Model file for the job. Use its own axes, mm. Coordinates: 2 decimals unless noted, no trailing zeros. Order: outer loops, then holes, each group sorted by start corner. A loop starts at its lowest first (then second) coordinate and runs counter-clockwise, first axis right, second up. Notation, with made-up numbers: M 83,-32 L 124,-32 A18 cw 124,-16 Z; hole C -1,-13.75 d10. An arc over 180 degrees is marked long. Return JSON: item names as keys, results as strings.
```python
from build123d import *

# Parameters (mm, degrees)
SKETCH1_W           = 12.7
SKETCH1_H           = 80
BOSS_EXTRUDE1_DEPTH = 12.7
SKETCH2_R           = 2.5
SKETCH2_R_2         = 2
CUT_EXTRUDE1_DEPTH  = 13.7


with BuildPart() as part:
    # Sketch1 → Boss-Extrude1 (new body)
    with BuildSketch(Plane.XY):
        with Locations((6.35, 40)):
            Rectangle(SKETCH1_W, SKETCH1_H)
    extrude(amount=BOSS_EXTRUDE1_DEPTH)

    # Sketch2 → Cut-Extrude1 (cut, through all)
    with BuildSketch(Plane.XY):
        with Locations((6.35, 5)):
            Circle(SKETCH2_R)
        with Locations((6.35, 20)):
            Circle(SKETCH2_R)
        with Locations((6.35, 60)):
            Circle(SKETCH2_R_2)
        with Locations((6.35, 75)):
            Circle(SKETCH2_R_2)
    extrude(amount=CUT_EXTRUDE1_DEPTH, mode=Mode.SUBTRACT)


solid = part.part
```
Item 1: Saw through at A-A (y = 60). Write the cut outline in (x, z).
Check result:
{"outline": "M 0,0 L 4.35,0 L 4.35,12.7 L 0,12.7 Z; M 8.35,0 L 12.7,0 L 12.7,12.7 L 8.35,12.7 Z"}
Item 2: Saw through at B-B (z = 8.75). Write the cut outline in (x, y), and give its area (3 significant figures).
Check result:
{"outline": "M 0,0 L 12.7,0 L 12.7,80 L 0,80 Z; hole C 6.35,5 d5; hole C 6.35,20 d5; hole C 6.35,60 d4; hole C 6.35,75 d4", "area": "952 mm2"}
Item 3: Pull direction Y, two halves, no side cores. Call faces 1 (the flat face through (6, 41, 12.7)), 2 (the flat face through (6, 80, 6)), 3 (the cylindrical face through (6.02, 22.48, 6.26)): +Y half, -Y half, draft (parallel to the pull), parting line (faces both ways), or undercut.
Check result:
{"face 1": "draft", "face 2": "+Y half", "face 3": "undercut"}
Item 4: Saw through at C-C (x = 6.35). Write the cut outline in (y, z).
Check result:
{"outline": "M 0,0 L 2.5,0 L 2.5,12.7 L 0,12.7 Z; M 7.5,0 L 17.5,0 L 17.5,12.7 L 7.5,12.7 Z; M 22.5,0 L 58,0 L 58,12.7 L 22.5,12.7 Z; M 62,0 L 73,0 L 73,12.7 L 62,12.7 Z; M 77,0 L 80,0 L 80,12.7 L 77,12.7 Z"}
Item 5: Saw through at D-D (y = 20). Write the cut outline in (x, z).
Check result:
{"outline": "M 0,0 L 3.85,0 L 3.85,12.7 L 0,12.7 Z; M 8.85,0 L 12.7,0 L 12.7,12.7 L 8.85,12.7 Z"}
Item 6: Wall check: line 1 (Y direction, x = 6.35, z = 7.5); line 2 (X direction, y = 60, z = 7.25); line 3 (X direction, y = 5, z = 10.25). Give the ranges that are in metal, low to high.
Check result:
{"line 1": "y = 0 to 2.5, 7.5 to 17.5, 22.5 to 58, 62 to 73, 77 to 80", "line 2": "x = 0 to 4.35, 8.35 to 12.7", "line 3": "x = 0 to 3.85, 8.85 to 12.7"}
